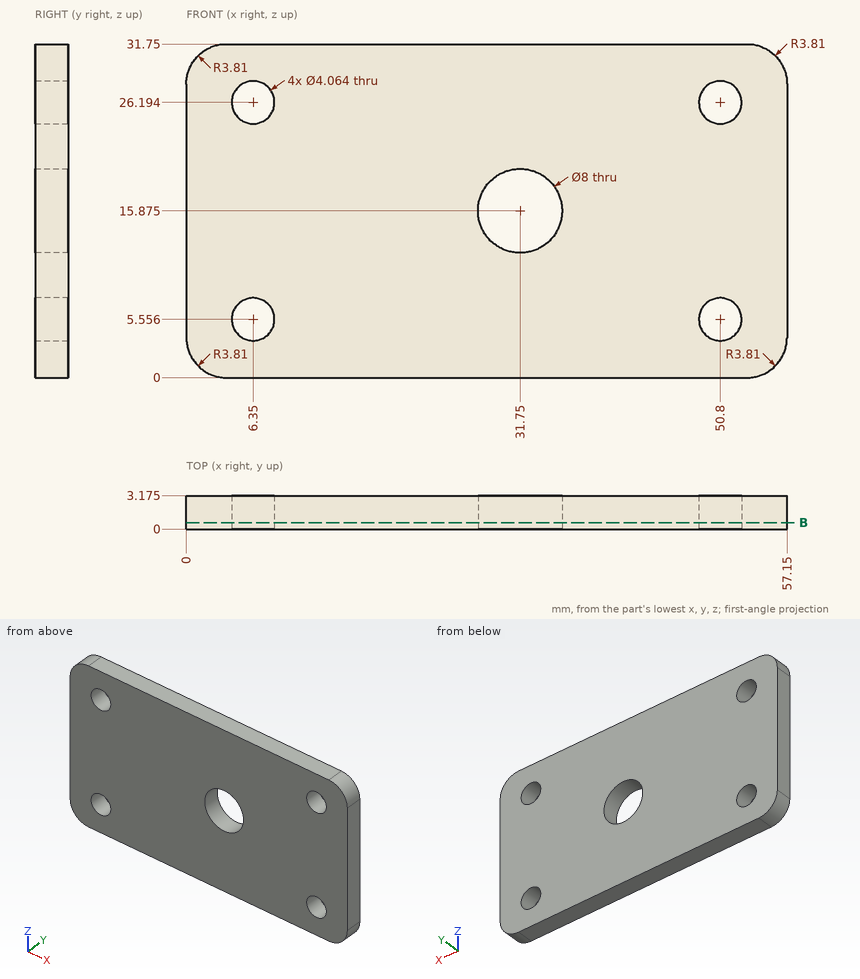
Input: dimensioned drawing with shaded views. Units: mm. Origin: part minimum x, y, z. Coordinates: 2 decimals unless noted, no trailing zeros. Put each result on its own line as item: value.
(1) Material intervals for probe 1 along X at (y, z) = (1.45, 25.5); probe 2 along Z at (x, y) = (8, 0.45); probe 3 along X at (y, z) = (2.7, 14), sorted ascending.
Answer sheet:
probe 1: x = 0 to 4.44, 8.26 to 48.89, 52.71 to 57.15
probe 2: z = 0 to 4.37, 6.74 to 25.01, 27.38 to 31.75
probe 3: x = 0 to 28.22, 35.28 to 57.15
(2) Cut plane B-B on y = 0.6. State how many separate pieces and enclosed holes the cut face has, then the cut area to 3 significant figures.
Answer sheet:
separate pieces: 1
enclosed holes: 5
area: 1,700 mm^2
(3) First-contact query: pin 1 (10.5 mm diameter, centred on x = 31.75, z = 15.875, fed in from -Y); pin 2 (3.5 mm diameter, centred on x = 50.8, z = 5.56, fed in from -Y). Flat tips, straight axial feed; report the tip coordinate or a pass-through.
Answer sheet:
pin 1: stops at y = 0
pin 2: passes through
